Check sheet for the modelled part. Datum: model origin and axes. Units: mm. A direction names the side the tool comes from. Round coordinates to 2 decimals unless told otherwise and drop trailing zeros. Order: outer loops, then holes, each group sorted by start corner. A loop starts at its lowest first (then second) coordinate and runs counter-clockwise, first axis right, second up. Notation, with made-up numbers: (70, 17.5) -> (93, 17.5) arc R23 cw to (93, 42.5) -> close; hole circle Ø9 at (60.5, 38.25). An arc over 180 degrees is marked (long way). Answer as CSV lines item,"result". Start each with the question number.
from build123d import *

# Parameters (mm, degrees)
SCHIZZO1_R                   = 2
ESTRUSIONE_ESTRUSIONE1_DEPTH = 4
RACCORDO1_R                  = 7
RACCORDO2_R                  = 5
RACCORDO3_R                  = 10
RACCORDO4_R                  = 2


with BuildPart() as part:
    # Schizzo1 → Estrusione-Estrusione1 (new body)
    with BuildSketch(Plane.XY):
        Polygon((0, 0), (0, 70), (25, 70), (25, 20), (70, 30), (70, 0), align=None)
        with Locations((12.5, 11.4)):
            Circle(SCHIZZO1_R, mode=Mode.SUBTRACT)
        with Locations((12.5, 54.6)):
            Circle(SCHIZZO1_R, mode=Mode.SUBTRACT)
        with Locations((61.5, 14.9)):
            Circle(SCHIZZO1_R, mode=Mode.SUBTRACT)
    extrude(amount=ESTRUSIONE_ESTRUSIONE1_DEPTH)

    # Raccordo1
    raccordo1_edges = [part.edges().sort_by_distance(p)[0] for p in [
        (0, 70, 2),
        (25, 70, 2),
    ]]
    fillet(raccordo1_edges, radius=RACCORDO1_R)

    # Raccordo2
    raccordo2_edges = [part.edges().sort_by_distance(p)[0] for p in [
        (0, 0, 2),
        (70, 0, 2),
    ]]
    fillet(raccordo2_edges, radius=RACCORDO2_R)

    # Raccordo3
    raccordo3_edges = [part.edges().sort_by_distance(p)[0] for p in [
        (70, 30, 2),
    ]]
    fillet(raccordo3_edges, radius=RACCORDO3_R)

    # Raccordo4
    raccordo4_edges = [part.edges().sort_by_distance(p)[0] for p in [
        (25, 20, 2),
    ]]
    fillet(raccordo4_edges, radius=RACCORDO4_R)


solid = part.part
1) Section check A-A on y = 14.9. Record the cut outline in (x, z).
2) Section check B-B on z = 2.6. Record the cut outline in (x, y).
3) Section check D-D on x = 61.5. Record the cut outline in (y, z), then the cut area to 3 significant figures.
4) Mould release check, pull along Y, two halves, no side actions. Record for faces 3 (the face through (12.066, 52.648, 1.972)), 4 (the face through (12.066, 9.448, 1.972)), 5 (the face through (0, 34, 2)), 6 (the face through (68, 1, 2)): released by +Y, released by -Y, zero draft, split by the parting line, or undercut.
5) Section check C-C on x = 12.5. Record the cut outline in (y, z), then the cut area to 3 significant figures.
6) Access from +Z, -Z, +X, -X, +Y, -Y to the whole of each face (thin tool, end or side, straight path). Record for faces 1 (the face through (42.42, 23.87, 1.97)), 2 (the face through (35, 0, 2)).
7) Material ranges on line 1 along Y through (x, z) = (12.5, 2.35); line 2 along Y through (x, z) = (11, 1.4); line 3 along X through (y, z) = (41, 0.2), recorded low to high.
8) Depth check by flat-ended pin: pin 1 Ø1 at (x, y) = (13, 24) entering from -Z; pin 2 Ø1 at (y, z) = (43.5, 0.5) entering from +X; pin 3 Ø1 at (y, z) = (25, 1) entering from +X. Enter the tip coordinate at first touch or a pass-through.
Solutions:
1,outline,"(0, 0) -> (59.5, 0) -> (59.5, 4) -> (0, 4) -> close; (63.5, 0) -> (70, 0) -> (70, 4) -> (63.5, 4) -> close"
2,outline,"(0, 5) arc R5 ccw to (5, 0) -> (65, 0) arc R5 ccw to (70, 5) -> (70, 17.53) arc R10 ccw to (57.83, 27.3) -> (27.43, 20.54) arc R2 cw to (25, 22.49) -> (25, 63) arc R7 ccw to (18, 70) -> (7, 70) arc R7 ccw to (0, 63) -> close; hole circle Ø4 at (12.5, 11.4); hole circle Ø4 at (12.5, 54.6); hole circle Ø4 at (61.5, 14.9)"
3,outline,"(0, 0) -> (12.9, 0) -> (12.9, 4) -> (0, 4) -> close; (16.9, 0) -> (27.42, 0) -> (27.42, 4) -> (16.9, 4) -> close"
3,area,"93.7 mm^2"
4,face 3,"undercut"
4,face 4,"undercut"
4,face 5,"zero draft"
4,face 6,"released by -Y"
5,outline,"(0, 0) -> (9.4, 0) -> (9.4, 4) -> (0, 4) -> close; (13.4, 0) -> (52.6, 0) -> (52.6, 4) -> (13.4, 4) -> close; (56.6, 0) -> (70, 0) -> (70, 4) -> (56.6, 4) -> close"
5,area,"248 mm^2"
6,face 1,"+Z, -Z, +Y"
6,face 2,"+Z, -Z, +X, -X, -Y"
7,line 1,"y = 0 to 9.4, 13.4 to 52.6, 56.6 to 70"
7,line 2,"y = 0 to 10.08, 12.72 to 53.28, 55.92 to 70"
7,line 3,"x = 0 to 25"
8,pin 1,"stops at z = 0"
8,pin 2,"stops at x = 25"
8,pin 3,"stops at x = 67.17"
